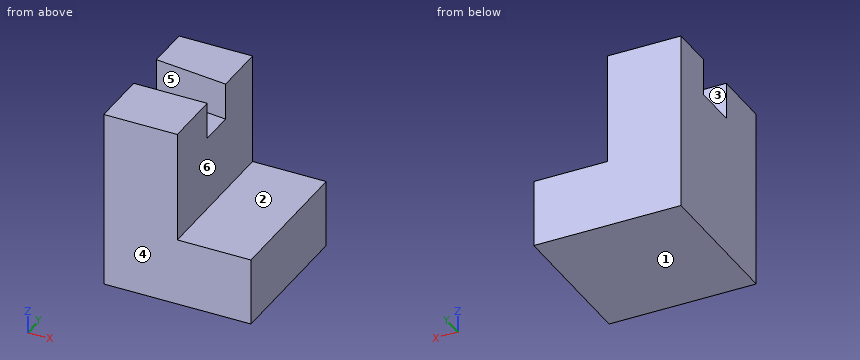
from build123d import *

# Parameters (mm, degrees)
F0_W     = 38.1
F0_H     = 30.7473719984
F1_DEPTH = 25.4
F2_W     = 25.4
F2_H     = 19.1348433927
F3_DEPTH = 12.7
F4_W     = 12.7244254082
F4_H     = 30.7473719984
F5_DEPTH = 25.4
F7_DEPTH = 6.35


with BuildPart() as f1:
    # F0 (on Front) → F1 (new body)
    with BuildSketch(Plane.XZ):
        with Locations((-37.9534605891, 41.5436550975)):
            Rectangle(F0_W, F0_H)
    extrude(amount=F1_DEPTH)

    # F2 (on face) → F3 (cut)
    with BuildSketch(Plane.YZ.offset(-18.9034605891)):
        with Locations((-12.7, 47.3499194004)):
            Rectangle(F2_W, F2_H)
    extrude(amount=-F3_DEPTH, mode=Mode.SUBTRACT)

    # F4 (on face) → F5 (cut)
    with BuildSketch(Plane(origin=(0, 0, 0), x_dir=(-1, 0, 0), z_dir=(0, 1, 0))):
        with Locations((50.6412478849, 41.5436550975)):
            Rectangle(F4_W, F4_H)
    extrude(amount=-F5_DEPTH, mode=Mode.SUBTRACT)

    # F6 (on face) → F7 (cut)
    with BuildSketch(Plane.XY.offset(56.9173410967)):
        Polygon((-44.2790351808, -7.6469713822), (-44.2790351808, -15.3137892485), (-31.6034605891, -15.3137892485), (-31.6034605891, -9.0938359499), align=None)
    extrude(amount=-F7_DEPTH, mode=Mode.SUBTRACT)


solid = f1.part
Model file for the job. Use its own axes, mm. Face numbers are marked on the shaded views. A direction names the side the tool comes from. Round coordinates to 2 decimals unless told otherwise and drop trailing zeros. Order: outer loops, then holes, each group sorted by start corner. A loop starts at its lowest first (then second) coordinate and runs counter-clockwise, first axis right, second up. Notation, with made-up numbers: M 22,81.5 L 68,81.5 A17 cw 68,113.5 Z; hole C 12.25,62 d11. An arc over 180 degrees is marked long. Write each question's results on one line, items separated by ' | '. Start each with the question number.
(1) Probe probe 1 along Z at (x, y) = (-39.25, -13.5); probe 2 along Z at (x, y) = (-25.75, -15.25); probe 3 along X at (y, z) = (-4, 45.5). List the from-to ranges inside material, lowest first. Write a range as from..to.
(2) Drop flat-ended pins along their axis: pin 1 (2.5 mm diameter, centred on x = -37.5, y = -13, fed in from +Z); pin 2 (4 mm diameter, centred on x = -25.5, y = -11.5, fed in from +Z); pin 3 (12 mm diameter, centred on y = -5.5, z = 47, fed in from +X). Give the stop position or say it passes through.
(3) Saw through at C-C, the plane z = 43. Give the cut face in (x, y), then the cut area to 3 significant figures.
(4) Two-plate mould, pull along Y, no slides. Class the marked faces 4, 5 and 6: pulls with the +Y half, pulls with the -Y half, needs draft (parallel to the pull), parting line crosses it, or undercut.
(5) Which spindle directions (+Z, -Z, +X, -X, +Y, -Y) get a long thin tool onto all of the face, cutting with end or side? Do the marked faces 1, 2 and 3. Say none if no direction does.
(6) Saw through at A-A, the plane y = -9.5. Give the cut face in (x, z).
(7) Saw through at D-D, the plane y = -17. Give the cut face in (x, z), then the cut area to 3 significant figures.
(8) Saw through at B-B, the plane x = -35. Give the cut face in (y, z), then the cut area to 3 significant figures.
Established:
1) probe 1: z = 26.17..50.57 | probe 2: z = 26.17..37.78 | probe 3: x = -44.28..-31.6
2) pin 1: stops at z = 50.57 | pin 2: stops at z = 37.78 | pin 3: stops at x = -31.6
3) outline: M -44.28,-25.4 L -31.6,-25.4 L -31.6,0 L -44.28,0 Z | area: 322 mm^2
4) face 4: pulls with the -Y half | face 5: undercut | face 6: needs draft
5) face 1: -Z, +X, -X, +Y, -Y | face 2: +Z, +X, +Y, -Y | face 3: +Z, +X, -X
6) outline: M -44.28,26.17 L -18.9,26.17 L -18.9,37.78 L -31.6,37.78 L -31.6,50.57 L -44.28,50.57 Z
7) outline: M -44.28,26.17 L -18.9,26.17 L -18.9,37.78 L -31.6,37.78 L -31.6,56.92 L -44.28,56.92 Z | area: 537 mm^2
8) outline: M -25.4,26.17 L 0,26.17 L 0,56.92 L -8.71,56.92 L -8.71,50.57 L -15.31,50.57 L -15.31,56.92 L -25.4,56.92 Z | area: 739 mm^2
